from build123d import *

# Parameters (mm, degrees)
FILLET1_R    = 0.1
SKETCH3_W    = 0.48
SKETCH3_H    = 1.6
SKETCH4_W    = 0.48
SKETCH4_H    = 0.702553256
RECPAT_COUNT = 2
RECPAT_ANGLE = 90


with BuildPart() as part:
    # BodySke → Base-Revolve (revolve)
    with BuildSketch(Plane.XY):
        with BuildLine():
            Line((1.3, 0.8), (1.3, 1.6))
            Line((1.3, 1.6), (0.650675799, 1.6))
            ThreePointArc((0.650675799, 1.6), (0.585036553, 1.584875829), (0.532633829, 1.542553191))
            ThreePointArc((0.532633829, 1.542553191), (0.136907172, 0.815960959), (0, 0))
            Line((0, 0), (9.3, 0))
            Line((9.3, 0), (9.3, 0.8))
            Line((9.3, 0.8), (1.3, 0.8))
        make_face()
    revolve(axis=Axis((-25.4, 0, 0), (1, 0, 0)))

    # Fillet1
    fillet1_edges = [part.edges().sort_by_distance(p)[0] for p in [
        (1.3, -0.8, 0),
    ]]
    fillet(fillet1_edges, radius=FILLET1_R)

    # Sketch3 → Recess section 0
    with BuildSketch(Plane(origin=(0, 0, 0), x_dir=(0, 0, -1), z_dir=(1, 0, 0))):
        Rectangle(SKETCH3_W, SKETCH3_H)
    # Sketch4 → Recess section 1
    with BuildSketch(Plane(origin=(0.9, 0, 0), x_dir=(0, 0, -1), z_dir=(1, 0, 0))):
        Rectangle(SKETCH4_W, SKETCH4_H)
    recess = loft(mode=Mode.SUBTRACT)

    # RecPat: Recess ×2 about axis
    recpat_axis = Axis((0, 0, 0), (1, 0, 0))
    for i in range(1, RECPAT_COUNT):
        add(recess.rotate(recpat_axis, i * RECPAT_ANGLE / (RECPAT_COUNT - 1)), mode=Mode.SUBTRACT)

    # RecCorSke → RecessCore (revolve, cut)
    with BuildSketch(Plane.XY):
        Polygon((0, 0), (0, 0.418434131), (0.9, 0.3555), (1.015508952, 0), align=None)
    revolve(axis=Axis((-3.175, 0, 0), (1, 0, 0)), mode=Mode.SUBTRACT)


solid = part.part
Part model, mm, in its own coordinate system. A direction names the side the tool comes from. Give positions to 0.01 mm unless a question says otherwise; leave off trailing zeros. Loops run counter-clockwise (first coordinate to the right, second up) from the corner with the lowest first, then second, coordinate; pieces in that order, holes last. Notation, with made-up numbers: M 78.25,-4.5 L 121.25,-4.5 A32 ccw 121.25,34.5 Z; hole C 80.5,-31 d11. An arc over 180 degrees is marked long. Put each result on its own line as item: value. Start each with the question number.
1) Saw through at A-A (x = 2). List the corners of the cut face in (y, z).
2) Probe probe 1 along Y at (x, z) = (4.5, 0.6); probe 2 along Z at (x, y) = (0.5, -0.2); probe 3 along X at (y, z) = (0.15, 1.2). List the from-to ranges inside material, lowest first.
3) 3-axis set-ups, long thin cutter, end or side, ignore diameter. For faces 1 (the cylindrical face through (5.29, -0.63, -0.49)), 2 (the flat face through (9.3, 0, 0)): which of +Z, -Z, +X, -X, +Y, -Y reach the whole face in a straight line?
4) Flat gauge pin, fed straight in: pin 1 (1.5 mm diameter, centred on y = -1, z = -0.5, fed in from +X). Where does the tip first touch, or does it go through?
Numbers:
1. outline: C 0,0 d1.6
2. probe 1: -0.53 to 0.53
2. probe 2: -1.49 to -0.55, 0.55 to 1.49
2. probe 3: 0.31 to 1.3
3. face 1: +X
3. face 2: +Z, -Z, +X, +Y, -Y
4. pin 1: x = 9.3
